CAD build for the part. Positions are in the model's coordinates, mm. Round coordinates to 2 decimals unless told otherwise and drop trailing zeros. Write each loop counter-clockwise with the first axis right and the second up, starting at its lowest first coordinate (ties: lowest second). Pieces come first, ordered by that corner, then holes. Notation, with made-up numbers: (-1, 17) - (19, 17) arc R4 cw to (19, 23) - close; hole circle Ø3 at (17.5, -5). An arc over 180 degrees is marked (long way). Answer in a Markdown table with one row per item.
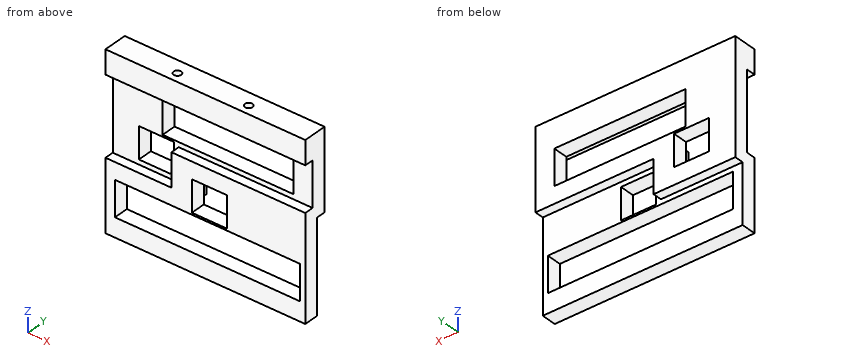
```python
from build123d import *

# Parameters (mm, degrees)
SKETCH1_W                 = 210.4
SKETCH1_H                 = 181.5
SKETCH1_W_2               = 138
SKETCH1_H_2               = 37
SKETCH1_W_3               = 37
SKETCH1_H_3               = 33
SKETCH1_W_4               = 195
BOSS_EXTRUDE1_DEPTH       = 25
SKETCH2_W                 = 37
SKETCH2_H                 = 33
SKETCH2_W_2               = 195
SKETCH2_H_2               = 37
CUT_EXTRUDE1_DEPTH        = 282.126821915
CUT_EXTRUDE1_DEPTH_BACK   = 9.5
SKETCH3_W                 = 37
SKETCH3_H                 = 33
SKETCH3_W_2               = 138
SKETCH3_H_2               = 37
CUT_EXTRUDE2_DEPTH        = 282.126821915
CUT_EXTRUDE2_DEPTH_BACK   = 9.5
F_8_0MM_DOWEL_HOLE1_D     = 8
F_8_0MM_DOWEL_HOLE1_DEPTH = 25


with BuildPart() as part:
    # Sketch1 → Boss-Extrude1 (new body)
    with BuildSketch(Plane(origin=(0, 0, 0), x_dir=(1, 0, 0), z_dir=(0, 1, 0))):
        with Locations((0, 168.75)):
            Rectangle(SKETCH1_W, SKETCH1_H)
        with Locations((16.3, 126.5)):
            Rectangle(SKETCH1_W_2, SKETCH1_H_2, mode=Mode.SUBTRACT)
        with Locations((-59.2, 163.5)):
            Rectangle(SKETCH1_W_3, SKETCH1_H_3, mode=Mode.SUBTRACT)
        with Locations((4.3, 184)):
            Rectangle(SKETCH1_W_3, SKETCH1_H_3, mode=Mode.SUBTRACT)
        with Locations((2.3, 221)):
            Rectangle(SKETCH1_W_4, SKETCH1_H_2, mode=Mode.SUBTRACT)
    extrude(amount=BOSS_EXTRUDE1_DEPTH)

    # Sketch2 → Cut-Extrude1 (cut, two sides)
    with BuildSketch(Plane(origin=(0, 25, 0), x_dir=(1, 0, 0), z_dir=(0, 1, 0))) as cut_extrude1_sk:
        Polygon((-105.2, 259.5), (-105.2, 197.5), (-19.2, 197.5), (-19.2, 162.5), (105.2, 162.5), (105.2, 259.5), align=None)
        with Locations((4.3, 184)):
            Rectangle(SKETCH2_W, SKETCH2_H, mode=Mode.SUBTRACT)
        with Locations((2.3, 221)):
            Rectangle(SKETCH2_W_2, SKETCH2_H_2, mode=Mode.SUBTRACT)
    extrude(amount=CUT_EXTRUDE1_DEPTH, mode=Mode.SUBTRACT)
    extrude(cut_extrude1_sk.sketch, amount=-CUT_EXTRUDE1_DEPTH_BACK, mode=Mode.SUBTRACT)

    # Sketch3 → Cut-Extrude2 (cut, two sides)
    with BuildSketch(Plane.XZ) as cut_extrude2_sk:
        Polygon((-105.2, -103), (-105.2, -185), (-35.7, -185), (-35.7, -150), (105.2, -150), (105.2, -103), align=None)
        with Locations((-59.2, -163.5)):
            Rectangle(SKETCH3_W, SKETCH3_H, mode=Mode.SUBTRACT)
        with Locations((16.3, -126.5)):
            Rectangle(SKETCH3_W_2, SKETCH3_H_2, mode=Mode.SUBTRACT)
    extrude(amount=CUT_EXTRUDE2_DEPTH, mode=Mode.SUBTRACT)
    extrude(cut_extrude2_sk.sketch, amount=-CUT_EXTRUDE2_DEPTH_BACK, mode=Mode.SUBTRACT)

    # Ø8.0mm Dowel Hole1
    with Locations(Plane(origin=(-37.5, 10, -78), x_dir=(1, 0, 0), z_dir=(0, 0, 1))):
        with Locations((0, 0), (75, 0)):
            Hole(F_8_0MM_DOWEL_HOLE1_D / 2, depth=F_8_0MM_DOWEL_HOLE1_DEPTH)


solid = part.part
```
Q1. Saw through at D-D on z = -208. List the corners of the cut face in (x, y), then the cut area to 3 significant figures.
Computed:
| item | result |
|---|---|
| outline | (-105.2, 0) - (-95.2, 0) - (-95.2, 15.5) - (-105.2, 15.5) - close; (99.8, 0) - (105.2, 0) - (105.2, 15.5) - (99.8, 15.5) - close |
| area | 239 mm2 |
Q2. Saw through at B-B on y = 3.5. List the corners of the cut face in (x, z), then the cut area to 3 significant figures.
Computed:
| item | result |
|---|---|
| outline | (-105.2, -259.5) - (105.2, -259.5) - (105.2, -150) - (-35.7, -150) - (-35.7, -185) - (-105.2, -185) - close; (-105.2, -103) - (105.2, -103) - (105.2, -78) - (-105.2, -78) - close; hole (-95.2, -239.5) - (99.8, -239.5) - (99.8, -202.5) - (-95.2, -202.5) - close; hole (-14.2, -200.5) - (22.8, -200.5) - (22.8, -167.5) - (-14.2, -167.5) - close |
| area | 17,400 mm2 |
Q3. Drill centre lines: line 1 (X direction, y = 10, z = -96); line 2 (Z direction, x = -62.5, y = 3.75); line 3 (Z direction, x = 16, y = 9). Where is each one in solid material? Low to high.
Computed:
| item | result |
|---|---|
| line 1 | x = -105.2 to -41.5, -33.5 to 33.5, 41.5 to 105.2 |
| line 2 | z = -259.5 to -239.5, -202.5 to -185, -103 to -78 |
| line 3 | z = -259.5 to -239.5, -202.5 to -200.5, -167.5 to -150, -103 to -78 |
Q4. Saw through at A-A on x = -85. List the corners of the cut face in (y, z), then the cut area to 3 significant figures.
Computed:
| item | result |
|---|---|
| outline | (0, -259.5) - (15.5, -259.5) - (15.5, -239.5) - (0, -239.5) - close; (0, -202.5) - (15.5, -202.5) - (15.5, -197.5) - (25, -197.5) - (25, -78) - (0, -78) - (0, -103) - (9.5, -103) - (9.5, -185) - (0, -185) - close |
| area | 2,600 mm2 |
Q5. Flat gauge pins, fed straight in: pin 1 (1 mm diameter, centred on x = 28.5, y = 20, fed in from -Z); pin 2 (1.5 mm diameter, centred on y = 4, z = -179, fed in from -X); pin 3 (10.5 mm diameter, centred on y = 21.5, z = -178, fed in from +X). Where does each tip first touch, or does it go through?
Computed:
| item | result |
|---|---|
| pin 1 | stops at z = -162.5 |
| pin 2 | stops at x = -35.7 |
| pin 3 | stops at x = -19.2 |
Q6. Saw through at C-C on x = 37.5. List the corners of the cut face in (y, z).
Computed:
| item | result |
|---|---|
| outline | (0, -259.5) - (15.5, -259.5) - (15.5, -239.5) - (0, -239.5) - close; (0, -202.5) - (15.5, -202.5) - (15.5, -162.5) - (25, -162.5) - (25, -145) - (9.5, -145) - (9.5, -150) - (0, -150) - close; (0, -103) - (6, -103) - (6, -78) - (0, -78) - close; (9.5, -108) - (25, -108) - (25, -78) - (14, -78) - (14, -103) - (9.5, -103) - close |
